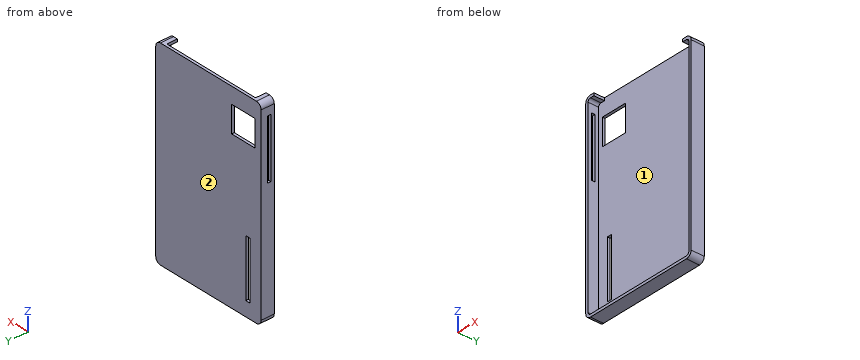
```python
from build123d import *

# Parameters (mm, degrees)
F0_W      = 114.3
F0_H      = 190.5
F1_DEPTH  = 12.7
F2_R      = 5.08
F3_T      = -2.54
F4_W      = 3.936436
F4_H      = 103.5833
F4_W_2    = 25.4
F4_H_2    = 25.4
F5_DEPTH  = 2.541
F6_W      = 3.333682
F6_H      = 57.772115
F7_DEPTH  = 2.541
F8_DEPTH  = 2.541
F9_W      = 96.21381
F9_H      = 10.16
F10_DEPTH = 2.541
F11_W     = 4.455637
F11_H     = 55.695463
F12_DEPTH = 2.541


with BuildPart() as f1:
    # F0 (on Front) → F1 (new body)
    with BuildSketch(Plane.XZ):
        with Locations((6.678557, 11.712478)):
            Rectangle(F0_W, F0_H)
    extrude(amount=F1_DEPTH)

    # F2
    f2_edges = [f1.edges().sort_by_distance(p)[0] for p in [
        (-50.471443, -6.35, 106.962478),
        (-50.471443, -6.35, -83.537522),
        (63.828557, -6.35, -83.537522),
        (63.828557, -6.35, 106.962478),
    ]]
    fillet(f2_edges, radius=F2_R)

    # F3
    f3_openings = [f1.faces().sort_by_distance(p)[0] for p in [
        (6.678557, -12.7, 11.712478),
    ]]
    offset(amount=F3_T, openings=f3_openings)

    # F4 (on face) → F5 (cut, through all)
    with BuildSketch(Plane.XZ.offset(2.54)):
        with Locations((-54.036425, 42.818326)):
            Rectangle(F4_W, F4_H)
        with Locations((-31.234852, 78.72139)):
            Rectangle(F4_W_2, F4_H_2)
    extrude(amount=-F5_DEPTH, mode=Mode.SUBTRACT)

    # F6 (on face) → F7 (cut, through all)
    with BuildSketch(Plane.YZ.offset(-47.931443)):
        with Locations((-7.72619, 65.276027)):
            Rectangle(F6_W, F6_H)
    extrude(amount=-F7_DEPTH, mode=Mode.SUBTRACT)

    # F4 (on face) → F8 (cut, through all)
    with BuildSketch(Plane.XZ.offset(2.54)):
        with Locations((-54.036425, 42.818326)):
            Rectangle(F4_W, F4_H)
        with Locations((-31.234852, 78.72139)):
            Rectangle(F4_W_2, F4_H_2)
    extrude(amount=-F8_DEPTH, mode=Mode.SUBTRACT)

    # F9 (on face) → F10 (cut, through all)
    with BuildSketch(Plane(origin=(0, 0, 104.422478), x_dir=(1, 0, 0), z_dir=(0, 0, -1))):
        with Locations((6.513808, 7.62)):
            Rectangle(F9_W, F9_H)
    extrude(amount=-F10_DEPTH, mode=Mode.SUBTRACT)

    # F11 (on face) → F12 (cut, through all)
    with BuildSketch(Plane.XZ.offset(2.54)):
        with Locations((-36.106074, -41.727004)):
            Rectangle(F11_W, F11_H)
    extrude(amount=-F12_DEPTH, mode=Mode.SUBTRACT)


solid = f1.part
```
Input: part model. Units: mm. Frame: model coordinates. Face numbers are marked on the shaded views. Give positions to 0.01 mm unless a question says otherwise; leave off trailing zeros. Order: outer loops, then holes, each group sorted by start corner. A loop starts at its lowest first (then second) coordinate and runs counter-clockwise, first axis right, second up. Notation, with made-up numbers: (63.25, 42.25) - (84.25, 42.25) arc R31 cw to (84.25, 73.25) - close; hole circle Ø3 at (25.5, 38). An arc over 180 degrees is marked (long way). Put each result on its own line as item: value.
Item 1: Section query A-A, the plane z = -20. Return loops of the section in (x, y), then the cut area to 3 significant figures.
Found:
outline: (-50.47, -12.7) - (-47.93, -12.7) - (-47.93, -2.54) - (-38.33, -2.54) - (-38.33, 0) - (-50.47, 0) - close; (-33.88, -2.54) - (61.29, -2.54) - (61.29, -12.7) - (63.83, -12.7) - (63.83, 0) - (-33.88, 0) - close
area: 331 mm^2
Item 2: Contact query for flat-ended pins moving along their axis: pin 1 (1.5 mm diameter, centred on y = -7, z = 81, fed in from -X); pin 2 (2 mm diameter, centred on x = -49, y = -7.5, fed in from +Z); pin 3 (0.8 mm diameter, centred on y = -5.5, z = 105.5, fed in from +X). Output: stop coordinate, or through.
Found:
pin 1: stops at x = 61.29
pin 2: stops at z = 106.24
pin 3: stops at x = 62.68
Item 3: Section query B-B, the plane x = -21.5. Return loops of the section in (y, z).
Found:
outline: (-12.7, -83.54) - (0, -83.54) - (0, 66.02) - (-2.54, 66.02) - (-2.54, -81) - (-12.7, -81) - close; (-2.54, 91.42) - (0, 91.42) - (0, 106.96) - (-2.54, 106.96) - close
Item 4: Draft query along X for the marked faces 1 and 2. Return one class per face: +X half, -X half, draft (parallel to the pull), parting line (faces both ways), or undercut.
Found:
face 1: undercut
face 2: draft
Item 5: Section query C-C, the plane z = 77. Return loops of the section in (x, y), then the cut area to 3 significant figures.
Found:
outline: (-50.47, -12.7) - (-47.93, -12.7) - (-47.93, -9.39) - (-50.47, -9.39) - close; (-50.47, -6.06) - (-47.93, -6.06) - (-47.93, -2.54) - (-43.93, -2.54) - (-43.93, 0) - (-50.47, 0) - close; (-18.53, -2.54) - (61.29, -2.54) - (61.29, -12.7) - (63.83, -12.7) - (63.83, 0) - (-18.53, 0) - close
area: 269 mm^2
Item 6: Section query D-D, the plane x = 11. Return loops of the section in (y, z).
Found:
outline: (-12.7, -83.54) - (0, -83.54) - (0, 106.96) - (-2.54, 106.96) - (-2.54, -81) - (-12.7, -81) - close
Item 7: Ray query, L1, parallel to X at y = -10.75, z = -13; L2, parallel to Z at x = -43.5, y = -0.5; L3, parallel to Y at x = -11.5, z = 63.5. Return the intervals inside material, ascending. Write a range as from..to.
Found:
L1: x = -50.47..-47.93, 61.29..63.83
L2: z = -83.54..66.02, 91.42..106.96
L3: y = -2.54..0
